```python
from build123d import *

# Parameters (mm, degrees)
SKETCH_1_R          = 1.5
EXTRUDE_1_DEPTH     = 5
SKETCH_2_R          = 1.5
CUT_EXTRUDE_4_DEPTH = 9
SKETCH1_R           = 2.5
CUT_EXTRUDE1_DEPTH  = 10


with BuildPart() as part:
    # Эскиз1 → Бобышка-Вытянуть1 (new body)
    # profile 1 of 2: a face of its own
    with BuildSketch(Plane(origin=(0, 0, 0), x_dir=(1, 0, 0), z_dir=(0, 1, 0))):
        with BuildLine():
            Line((0, 10), (0, 2))
            ThreePointArc((0, 2), (0.765366865, 1.847759065), (1.414213562, 1.414213562))
            Line((1.414213562, 1.414213562), (3.556747109, 3.556747109))
            ThreePointArc((3.556747109, 3.556747109), (3.556747109, 5.678067453), (5.678067453, 5.678067453))
            Line((5.678067453, 5.678067453), (7.071067812, 7.071067812))
            ThreePointArc((7.071067812, 7.071067812), (3.826834324, 9.238795325), (0, 10))
        make_face()
    # profile 2 of 2: a face of its own
    with BuildSketch(Plane(origin=(0, 0, 0), x_dir=(1, 0, 0), z_dir=(0, 1, 0))):
        with BuildLine():
            ThreePointArc((2, 0), (-1.414213562, -1.414213562), (0, 2))
            Line((0, 2), (0, 10))
            ThreePointArc((0, 10), (-7.071067812, -7.071067812), (10, 0))
            ThreePointArc((10, 0), (9.238795325, 3.826834324), (7.071067812, 7.071067812))
            Line((7.071067812, 7.071067812), (5.678067453, 5.678067453))
            ThreePointArc((5.678067453, 5.678067453), (6.00322658, 5.19143243), (6.117407281, 4.617407281))
            ThreePointArc((6.117407281, 4.617407281), (5.19143243, 3.231587982), (3.556747109, 3.556747109))
            Line((3.556747109, 3.556747109), (1.414213562, 1.414213562))
            ThreePointArc((1.414213562, 1.414213562), (1.847759065, 0.765366865), (2, 0))
        make_face()
        with Locations(Location((-4.617407281, -4.617407281, 0), (0, 0, 270))):
            Circle(SKETCH_1_R, mode=Mode.SUBTRACT)
        with Locations(Location((4.617407281, -4.617407281, 0), (0, 0, 270))):
            Circle(SKETCH_1_R, mode=Mode.SUBTRACT)
        with Locations(Location((-4.617407281, 4.617407281, 0), (0, 0, 270))):
            Circle(SKETCH_1_R, mode=Mode.SUBTRACT)
    extrude(amount=EXTRUDE_1_DEPTH)

    # Эскиз2 → Вырез-Вытянуть4 (cut)
    with BuildSketch(Plane(origin=(10, 0, 0), x_dir=(0, 0, -1), z_dir=(1, 0, 0))):
        with Locations((0, 2.5)):
            Circle(SKETCH_2_R)
    extrude(amount=-CUT_EXTRUDE_4_DEPTH, mode=Mode.SUBTRACT)

    # Sketch1 → Cut-Extrude1 (cut)
    with BuildSketch(Plane.XZ):
        with Locations(Location((0, 0, 0), (0, 0, 270))):
            Circle(SKETCH1_R)
    extrude(amount=-CUT_EXTRUDE1_DEPTH, mode=Mode.SUBTRACT)


solid = part.part
```
Model file for the job. Use its own axes, mm. Coordinates: 2 decimals unless noted, no trailing zeros. Loops run counter-clockwise (first coordinate to the right, second up) from the corner with the lowest first, then second, coordinate; pieces in that order, holes last. Notation, with made-up numbers: (89.5, 32.5) - (129.5, 32.5) arc R18 cw to (129.5, 62.5) - close; hole circle Ø9 at (-36, 57.25). An arc over 180 degrees is marked (long way). Answer as a JSON object with one key per item and string values. Group by question number.
(1) Cut at A-A (x = -1). Give the cut face in (y, z).
(2) Cut at D-D (x = 1.75). Give the cut face in (y, z).
(3) Cut at C-C (x = 5). Give the cut face in (y, z).
(4) Flat gauge pins, fed straight in: pin 1 (1 mm diameter, centred on x = -3, y = 2, fed in from +Z); pin 2 (2.5 mm diameter, centred on x = -4.62, z = -4.62, fed in from +Y); pin 3 (2 mm diameter, centred on x = -4, y = 2, fed in from +Z); pin 4 (1 mm diameter, centred on y = 3, z = 2, fed in from +X). Where does each tip first touch, or does it go through?
(5) Cut at B-B (y = 1.45). Give the cut face in (x, z).
(6) Probe line 1 along X through (y, z) = (2.4, -5.25); line 2 along X through (y, z) = (2.4, 3.25); line 3 along Z through (x, y) = (-5.5, 0.95). List the from-to ranges inside material, lowest first.
(7) Two-plate mould, pull along Z, no slides. Class faces 1 (the face through (2, 5, 2)), 2 (the face through (6, 1, 0)), 3 (the face through (4.04, 2.46, 6)): released by +Z, released by -Z, zero draft, split by the parting line, or undercut.
Geometry says:
{
 "1": {"outline": "(0, -9.95) - (5, -9.95) - (5, -2.29) - (0, -2.29) - close; (0, 2.29) - (5, 2.29) - (5, 9.95) - (0, 9.95) - close"},
 "2": {"outline": "(0, -9.85) - (5, -9.85) - (5, -1.79) - (0, -1.79) - close; (0, 1.79) - (5, 1.79) - (5, 9.85) - (0, 9.85) - close"},
 "3": {"outline": "(0, -8.66) - (5, -8.66) - (5, -6.07) - (0, -6.07) - close; (0, -3.17) - (5, -3.17) - (5, 3.17) - (0, 3.17) - close; (0, 6.07) - (5, 6.07) - (5, 8.66) - (0, 8.66) - close; hole circle Ø3 at (2.5, 0)"},
 "4": {"pin 1": "stops at z = 9.68", "pin 2": "passes through", "pin 3": "stops at z = 9.54", "pin 4": "stops at x = 9.89"},
 "5": {"outline": "(2.26, -1.07) arc R2.5 cw (long way) to (2.26, 1.07) - (9.94, 1.07) arc R10 ccw (long way) to (9.94, -1.07) - close; hole circle Ø3 at (-4.62, -4.62); hole circle Ø3 at (-4.62, 4.62); hole circle Ø3 at (4.62, -4.62); hole circle Ø3 at (4.62, 4.62)"},
 "6": {"line 1": "x = -8.51 to -5.98, -3.26 to 3.26, 5.98 to 8.51", "line 2": "x = -9.46 to -5.23, -4 to 4, 5.23 to 9.46", "line 3": "z = -8.35 to -5.83, -3.4 to 3.4, 5.83 to 8.35"},
 "7": {"face 1": "zero draft", "face 2": "undercut", "face 3": "undercut"}
}
